The model under review builds one solid part; all positions refer to its coordinate system, in mm. A direction names the side the tool comes from. Give positions to 0.01 mm unless a question says otherwise; leave off trailing zeros. Write each loop counter-clockwise with the first axis right and the second up, starting at its lowest first coordinate (ties: lowest second). Pieces come first, ordered by that corner, then holes.
from build123d import *

# Parameters (mm, degrees)
ESQUISSE1_R                 = 4
BOSS_EXTRU_1_DEPTH          = 10
CHANFREIN3_SIZE             = 4
CONG_2_R                    = 4
ESQUISSE3_R                 = 4
BOSS_EXTRU_2_DEPTH          = 2
ENL_V_START                 = -42
ENL_V_MAT_EXTRU_4_OUTLINE_R = 2.75
ENL_V_MAT_EXTRU_4_DEPTH     = 9.0952626
CONG_4_R                    = 4
ESQUISSE7_R                 = 2.75
ENL_V_MAT_EXTRU_5_DEPTH     = 8.5
ESQUISSE7_4_R               = 3.5
ESQUISSE7_4_R_2             = 2.75
ENL_V_MAT_EXTRU_8_DEPTH     = 1
ESQUISSE8_R                 = 3.5
ENL_V_MAT_EXTRU_9_DEPTH     = 1
ENL_V_START_2               = -1
ESQUISSE9_R                 = 3.5
ENL_V_MAT_EXTRU_10_DEPTH    = 1


# Read off the part's stored shape, not the designer's step: Enlèv. mat.-Extru.4
with BuildPart() as part:
    # Esquisse1 → Boss.-Extru.1 (new body)
    # profile 1 of 4: a face of its own
    with BuildSketch(Plane(origin=(0, 0, 0), x_dir=(1, 0, 0), z_dir=(0, 1, 0))):
        Polygon((-18, 6.5), (-18, 12), (-18, 13.5), (-13, 13.5), (0, 13.5), (0, 20), (-42, 20), (-42, 12), (-42, 0), (-42, -12), (-18, -12), align=None)
        with Locations(Location((-30, 0, 0), (0, 0, 270))):
            Circle(ESQUISSE1_R, mode=Mode.SUBTRACT)
    # profile 2 of 4: a face of its own
    with BuildSketch(Plane(origin=(0, 0, 0), x_dir=(1, 0, 0), z_dir=(0, 1, 0))):
        Polygon((0, 20), (0, 13.5), (13, 13.5), (18, 13.5), (18, 12), (18, 6.5), (18, -12), (42, -12), (42, 0), (42, 12), (42, 20), align=None)
        with Locations(Location((30, 0, 0), (0, 0, 270))):
            Circle(ESQUISSE1_R, mode=Mode.SUBTRACT)
    # profile 3 of 4: a face of its own
    with BuildSketch(Plane(origin=(0, 0, 0), x_dir=(1, 0, 0), z_dir=(0, 1, 0))):
        Polygon((-18, 13.5), (-18, 12), (-18, 6.5), (-13, 13.5), align=None)
    # profile 4 of 4: a face of its own
    with BuildSketch(Plane(origin=(0, 0, 0), x_dir=(1, 0, 0), z_dir=(0, 1, 0))):
        Polygon((18, 13.5), (13, 13.5), (18, 6.5), (18, 12), align=None)
    extrude(amount=BOSS_EXTRU_1_DEPTH)

    # Chanfrein3
    chanfrein3_edges = [part.edges().sort_by_distance(p)[0] for p in [
        (-18, 5, 12),
        (-42, 5, 12),
        (42, 5, 12),
        (18, 5, 12),
    ]]
    chamfer(chanfrein3_edges, length=CHANFREIN3_SIZE)

    # Congé2
    cong_2_edges = [part.edges().sort_by_distance(p)[0] for p in [
        (42, 5, 8),
        (22, 5, 12),
        (38, 5, 12),
        (18, 5, 8),
        (-22, 5, 12),
        (-38, 5, 12),
        (-42, 5, 8),
        (-18, 5, 8),
    ]]
    fillet(cong_2_edges, radius=CONG_2_R)

    # Esquisse3 → Boss.-Extru.2 (add)
    with BuildSketch(Plane.XZ):
        with Locations(Location((-30, 0, 0), (0, 0, 270))):
            Circle(ESQUISSE3_R)
        with Locations(Location((30, 0, 0), (0, 0, 90))):
            Circle(ESQUISSE3_R)
    extrude(amount=-BOSS_EXTRU_2_DEPTH)

    # Enlèv. mat.-Extru.4 outline → Enlèv. mat.-Extru.4 (cut)
    with BuildSketch(Plane.YZ.offset(ENL_V_START)):
        with Locations((5.5, 0)):
            Circle(ENL_V_MAT_EXTRU_4_OUTLINE_R)
    enl_v_mat_extru_4 = extrude(amount=ENL_V_MAT_EXTRU_4_DEPTH, mode=Mode.SUBTRACT)

    # Symétrie10: Enlèv. mat.-Extru.4 across plane
    add(enl_v_mat_extru_4.mirror(Plane(origin=(0, 0, 0), x_dir=(0, 0, 1), z_dir=(1, 0, 0))), mode=Mode.SUBTRACT)

    # Congé4
    cong_4_edges = [part.edges().sort_by_distance(p)[0] for p in [
        (-42, 5, -20),
        (42, 5, -20),
        (18, 5, -6.5),
        (13, 5, -13.5),
        (-13, 5, -13.5),
        (-18, 5, -6.5),
    ]]
    fillet(cong_4_edges, radius=CONG_4_R)

    # Esquisse7 → Enlèv. mat.-Extru.5 (cut)
    with BuildSketch(Plane.XZ):
        with Locations(Location((-35, -13, 0), (0, 0, 270))):
            Circle(ESQUISSE7_R)
        with Locations(Location((35, -13, 0), (0, 0, 270))):
            Circle(ESQUISSE7_R)
    extrude(amount=-ENL_V_MAT_EXTRU_5_DEPTH, mode=Mode.SUBTRACT)

    # Esquisse7<4> → Enlèv. mat.-Extru.8 (cut)
    # profile 1 of 2: a face of its own
    with BuildSketch(Plane.XZ):
        with Locations(Location((-35, -13, 0), (0, 0, 270))):
            Circle(ESQUISSE7_4_R)
        with Locations(Location((-35, -13, 0), (0, 0, 270))):
            Circle(ESQUISSE7_4_R_2, mode=Mode.SUBTRACT)
    # profile 2 of 2: a face of its own
    with BuildSketch(Plane.XZ):
        with Locations(Location((35, -13, 0), (0, 0, 270))):
            Circle(ESQUISSE7_4_R)
        with Locations(Location((35, -13, 0), (0, 0, 270))):
            Circle(ESQUISSE7_4_R_2, mode=Mode.SUBTRACT)
    extrude(amount=-ENL_V_MAT_EXTRU_8_DEPTH, mode=Mode.SUBTRACT)

    # Esquisse8 → Enlèv. mat.-Extru.9 (cut)
    with BuildSketch(Plane.ZY.offset(42)):
        with Locations((0, 5.5)):
            Circle(ESQUISSE8_R)
    extrude(amount=-ENL_V_MAT_EXTRU_9_DEPTH, mode=Mode.SUBTRACT)

    # Esquisse9 → Enlèv. mat.-Extru.10 (cut)
    with BuildSketch(Plane(origin=(42, 0, 0), x_dir=(0, 0, -1), z_dir=(1, 0, 0)).offset(ENL_V_START_2)):
        with Locations(Location((0, 5.5, 0), (0, 0, 180))):
            Circle(ESQUISSE9_R)
    extrude(amount=ENL_V_MAT_EXTRU_10_DEPTH, mode=Mode.SUBTRACT)


solid = part.part
1) Consider section C-C, the plane x = 30. Give the boundary of the cut face in (y, z).
2) Consider section A-A, the plane z = 0. State how many separate pieces and enclosed holes the cut face has, then the cut area to 3 significant figures.
3) To check wall thickness, follow probe 1 along X at (y, z) = (8, 5.5); probe 2 along Y at (x, z) = (41.55, 0); probe 3 along Y at (x, z) = (37.25, 0). State the ranges of each line that lie inside material, in increasing order.
4) Insertion check: pin 1 (4 mm diameter, centred on x = 35, z = -13, fed in from -Y); pin 2 (3 mm diameter, centred on x = 4, y = 3.5, fed in from +Z); pin 3 (3.5 mm diameter, centred on y = 5.5, z = 0, fed in from +X). Each pin has a flat end and moves straight along its axis. Give the tip position at first contact, or say it passes through.
5) Consider section B-B, the plane x = -35. Give the boundary of the cut face in (y, z).
6) The part is to be moulded in two halves that separate along X. For faces 6 (the cylindrical face through (-32.273, 4.698, -12.642)), 7 (the flat face through (30, 2, 0)), 8 (the flat face through (-40, 5, 10)), 9 (the flat face through (40, 5, 10)), say which applies: +X half, -X half, draft (parallel to the pull), parting line (faces both ways), or undercut.
7) Tool access review of faces 1 (the flat face through (-30, 2, 0)), 2 (the cylindrical face through (-12.8, 5.07, -13.04)), 3 (the cylindrical face through (37.01, 8.04, -1.05)), 4 (the flat face through (34, 1, -10)), 5 (the flat face through (-41, 3, 2)): name each direction out of +Z, -Z, +X, -X, +Y, -Y from which nothing blocks a thin tool from reaching the whole face with its end or side.
Answer block:
1. outline: (0, -20) - (10, -20) - (10, -4) - (2, -4) - (2, 4) - (10, 4) - (10, 12) - (0, 12) - close
2. separate pieces: 4
2. enclosed holes: 0
2. area: 261 mm2
3. probe 1: x = -42 to -18, 18 to 42
3. probe 2: y = 0 to 2, 9 to 10
3. probe 3: y = 0 to 2.75, 8.25 to 10
4. pin 1: stops at y = 8.5
4. pin 2: stops at z = -13.5
4. pin 3: stops at x = 26.4
5. outline: (0, -20) - (10, -20) - (10, 12) - (0, 12) - (0, -9.5) - (1, -9.5) - (1, -10.25) - (8.5, -10.25) - (8.5, -15.75) - (1, -15.75) - (1, -16.5) - (0, -16.5) - close; hole circle Ø5.5 at (5.5, 0)
6. face 6: undercut
6. face 7: undercut
6. face 8: -X half
6. face 9: +X half
7. face 1: +Y
7. face 2: +Z, +Y, -Y
7. face 3: +X
7. face 4: -Y
7. face 5: -X
